Check sheet for the drawn part. Datum: minimum x, y, z corner. Units: mm. A direction names the side the tool comes from. Give positions to 0.01 mm unless a question says otherwise; leave off trailing zeros. Loops run counter-clockwise (first coordinate to the right, second up) from the corner with the lowest first, then second, coordinate; pieces in that order, holes last. Notation, with made-up numbers: (-34.5, 18) - (23.5, 18) arc R19 cw to (23.5, 32) - close; hole circle Ø7 at (-14.5, 66). An arc over 180 degrees is marked (long way). Use one line per item in the form item = value.
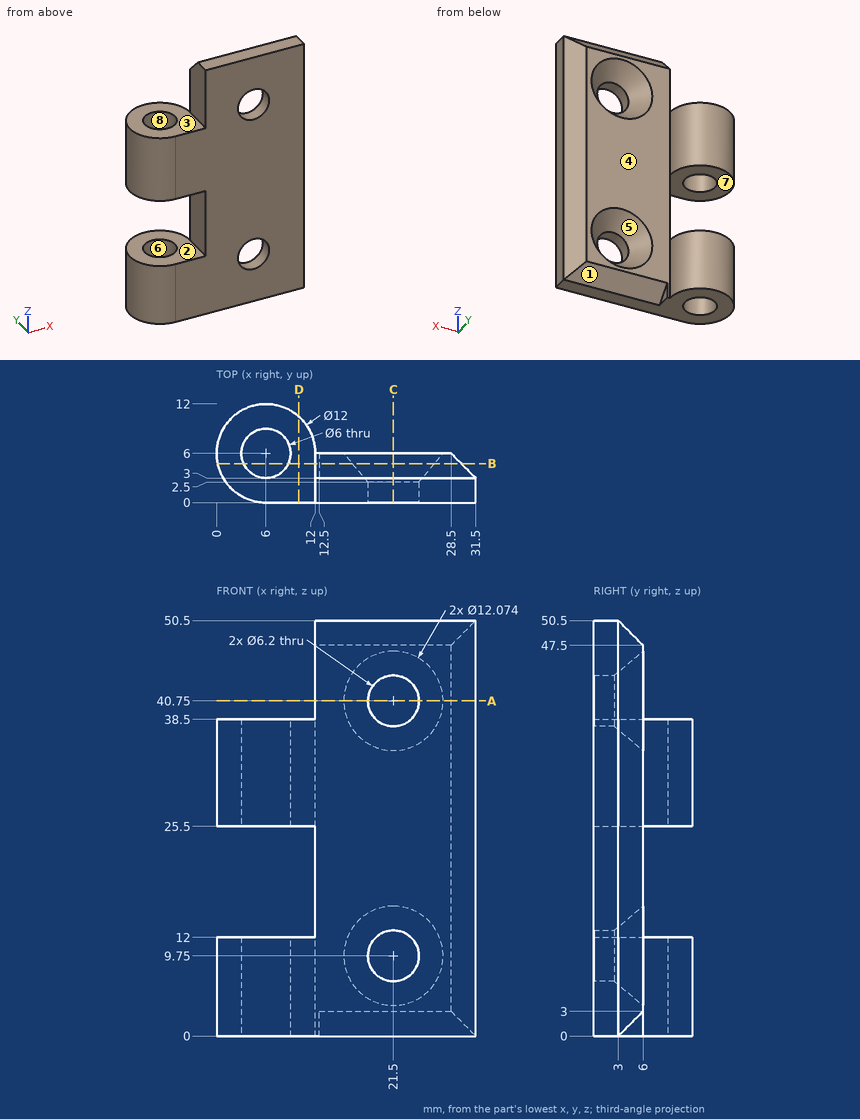
Item 1: Section check C-C on x = 21.5. Record the boundary of the cut face in (y, z).
Answer block:
outline = (0, 0) - (3, 0) - (6, 3) - (6, 3.71) - (2.5, 6.65) - (0, 6.65) - close; (0, 12.85) - (2.5, 12.85) - (6, 15.79) - (6, 34.71) - (2.5, 37.65) - (0, 37.65) - close; (0, 43.85) - (2.5, 43.85) - (6, 46.79) - (6, 47.5) - (3, 50.5) - (0, 50.5) - close
Item 2: Gauge pin test, flat ends, axial feed: P1, Ø5, axis at x = 17.5, z = 40.5, coming from the -Y side; P2, Ø6, axis at y = 1.5, z = 29, coming from the -X side; P3, Ø5.5, axis at x = 21.5, z = 40.75, coming from the -Y side; P4, Ø6.5, axis at y = 3.5, z = 45, coming from the -X side. Record the tip position at first contact, or that the pin passes through.
Answer block:
P1 = 0
P2 = 0.19
P3 = through
P4 = 12
Item 3: Mould release check, pull along Y, two halves, no side actions. Record for the marked faces 5, 6, 7 and 8: released by +Y, released by -Y, zero draft, split by the parting line, or undercut.
Answer block:
face_5 = released by +Y
face_6 = undercut
face_7 = zero draft
face_8 = undercut
Item 4: Section check D-D on x = 10. Record the boundary of the cut face in (y, z), then the cut area to 3 significant figures.
Answer block:
outline = (0, 0) - (10.47, 0) - (10.47, 12) - (0, 12) - close; (0, 25.5) - (10.47, 25.5) - (10.47, 38.5) - (0, 38.5) - close
area = 262 mm2
Item 5: Access from +Z, -Z, +X, -X, +Y, -Y to the whole of each face (thin tool, end or side, straight path). Record for the marked faces 1, 2, 3 and 4.
Answer block:
face_1 = -Z, +X, +Y
face_2 = -X, +Y, -Y
face_3 = +Z, -X, +Y, -Y
face_4 = +Z, -Z, +X, +Y
Item 6: Section check A-A on z = 40.75. Record the boundary of the cut face in (x, y).
Answer block:
outline = (12, 0) - (18.4, 0) - (18.4, 2.5) - (15.46, 6) - (12, 6) - close; (24.6, 0) - (31.5, 0) - (31.5, 3) - (28.5, 6) - (27.54, 6) - (24.6, 2.5) - close
Item 7: Section check B-B on y = 4.75. Record the boundary of the cut face in (x, z), then the cut area to 3 significant figures.
Answer block:
outline = (0.13, 0) - (3.27, 0) - (3.27, 12) - (0.13, 12) - close; (0.13, 25.5) - (3.27, 25.5) - (3.27, 38.5) - (0.13, 38.5) - close; (8.73, 0) - (12.5, 0) - (12.5, 1.75) - (29.75, 1.75) - (29.75, 48.75) - (12, 48.75) - (12, 38.5) - (8.73, 38.5) - (8.73, 25.5) - (12, 25.5) - (12, 12) - (8.73, 12) - close; hole circle Ø9.98 at (21.5, 9.75); hole circle Ø9.98 at (21.5, 40.75)
area = 839 mm2
Item 8: Thickness scan on L1, parallel to Z at x = 21.5, y = 1.75; L2, parallel to Y at x = 6, z = 34; L3, parallel to X at y = 4.5, z = 5.5 (1 decimal). Record the ranges inside material, lowest first.
Answer block:
L1 = 0 to 6.65, 12.85 to 37.65, 43.85 to 50.5
L2 = 0 to 3, 9 to 12
L3 = 0.2 to 3.4, 8.6 to 19.3, 23.7 to 30
